```python
from build123d import *

# Parameters (mm, degrees)
F_8_CLEARANCE_HOLE1_D = 4.4958


with BuildPart() as part:
    # Sketch1 → Revolve1 (revolve)
    with BuildSketch(Plane.XY):
        Polygon((-20.32, 7.62), (-20.32, 0), (-8.7503, 0), (-8.7503, 6.5278), (-10.2235, 6.5278), (-10.2235, 7.62), align=None)
    revolve(axis=Axis((0, 0, 0), (0, 1, 0)))

    # #8 Clearance Hole1 (through all)
    with Locations(Plane(origin=(0, 7.62, 0), x_dir=(1, 0, 0), z_dir=(0, 1, 0))):
        with Locations((13.97, 0), (0, 13.97), (-13.97, 0), (0, -13.97)):
            Hole(F_8_CLEARANCE_HOLE1_D / 2)


solid = part.part
```
Model file for the job. Use its own axes, mm. A direction names the side the tool comes from. Round coordinates to 2 decimals unless told otherwise and drop trailing zeros. Loops run counter-clockwise (first coordinate to the right, second up) from the corner with the lowest first, then second, coordinate; pieces in that order, holes last. Notation, with made-up numbers: M 82,-27.75 L 90,-27.75 A22 cw 90,-4.75 Z; hole C -7,63.5 d8. An arc over 180 degrees is marked long. Put each result on its own line as item: value. Start each with the question number.
Item 1: Cut at A-A (x = 0). List the corners of the cut face in (y, z), then the cut area to 3 significant figures.
Item 2: Drill centre lines: line 1 along Z through (x, y) = (0, 3); line 2 along Z through (x, y) = (0, 7.35); line 3 along Z through (x, y) = (15.5, 5). Where is each one in solid material? Low to high.
Item 3: Cut at C-C (z = 6). List the corners of the cut face in (x, y), then the cut area to 3 significant figures.
Item 4: Cut at D-D (y = 4.75). List the corners of the cut face in (x, z).
Item 5: Cut at B-B (z = 0). List the corners of the cut face in (x, y), then the cut area to 3 significant figures.
Item 6: Mould opens along X. For faces 1 (the face through (0, 0, -9)), 2 (the face through (2.645, 3.757, 20.147)), 3 (the face through (0.487, 3.757, -11.776)) say: released by +X, released by -X, zero draft, split by the parting line, or undercut.
Item 7: Drop flat-ended pins along their axis: P1, Ø1.5, axis at x = -14, y = 5, coming from the -Z side; P2, Ø16.5, axis at x = 0, z = 0, coming from the -Y side; P3, Ø3, axis at y = 4, z = 2, coming from the +X side; P4, Ø1, axis at x = 9, y = 2, coming from the -Z side. Give the stop position or say it passes through.
Item 8: 3-axis set-ups, long thin cutter, end or side, ignore diameter. For faces 4 (the face through (11.826, 3.757, -0.675)), 5 (the face through (8.113, 7.082, -6.221)): which of +Z, -Z, +X, -X, +Y, -Y reach the whole face in a straight line?
Answer block:
1. outline: M 0,-20.32 L 7.62,-20.32 L 7.62,-16.22 L 0,-16.22 Z; M 0,-11.72 L 7.62,-11.72 L 7.62,-10.22 L 6.53,-10.22 L 6.53,-8.75 L 0,-8.75 Z; M 0,8.75 L 6.53,8.75 L 6.53,10.22 L 7.62,10.22 L 7.62,11.72 L 0,11.72 Z; M 0,16.22 L 7.62,16.22 L 7.62,20.32 L 0,20.32 Z
1. area: 105 mm2
2. line 1: -20.32 to -16.22, -11.72 to -8.75, 8.75 to 11.72, 16.22 to 20.32
2. line 2: -20.32 to -16.22, -11.72 to -10.22, 10.22 to 11.72, 16.22 to 20.32
2. line 3: -13.14 to -1.65, 1.65 to 13.14
3. outline: M -19.41,0 L -6.37,0 L -6.37,6.53 L -8.28,6.53 L -8.28,7.62 L -19.41,7.62 Z; M 6.37,0 L 19.41,0 L 19.41,7.62 L 8.28,7.62 L 8.28,6.53 L 6.37,6.53 Z
3. area: 195 mm2
4. outline: C 0,0 d40.64; hole C -13.97,0 d4.5; hole C 0,0 d17.5; hole C 0,-13.97 d4.5; hole C 0,13.97 d4.5; hole C 13.97,0 d4.5
5. outline: M -20.32,0 L -16.22,0 L -16.22,7.62 L -20.32,7.62 Z; M -11.72,0 L -8.75,0 L -8.75,6.53 L -10.22,6.53 L -10.22,7.62 L -11.72,7.62 Z; M 8.75,0 L 11.72,0 L 11.72,7.62 L 10.22,7.62 L 10.22,6.53 L 8.75,6.53 Z; M 16.22,0 L 20.32,0 L 20.32,7.62 L 16.22,7.62 Z
5. area: 105 mm2
6. face 1: zero draft
6. face 2: split by the parting line
6. face 3: undercut
7. P1: z = -15.41
7. P2: through
7. P3: x = 20.31
7. P4: z = -18.46
8. face 4: +Y, -Y
8. face 5: +Y
